Drawing for the job (mm, zero at the part's lowest x, y, z). Coordinates: 2 decimals unless noted, no trailing zeros. Loops run counter-clockwise (first coordinate to the right, second up) from the corner with the lowest first, then second, coordinate; pieces in that order, holes last. Notation, with made-up numbers: (27.5, 85.25) - (69.5, 85.25) arc R11 cw to (69.5, 106.25) - close; hole circle Ø1 at (35.5, 35.5). An arc over 180 degrees is marked (long way). Put each result on its own line as item: value.
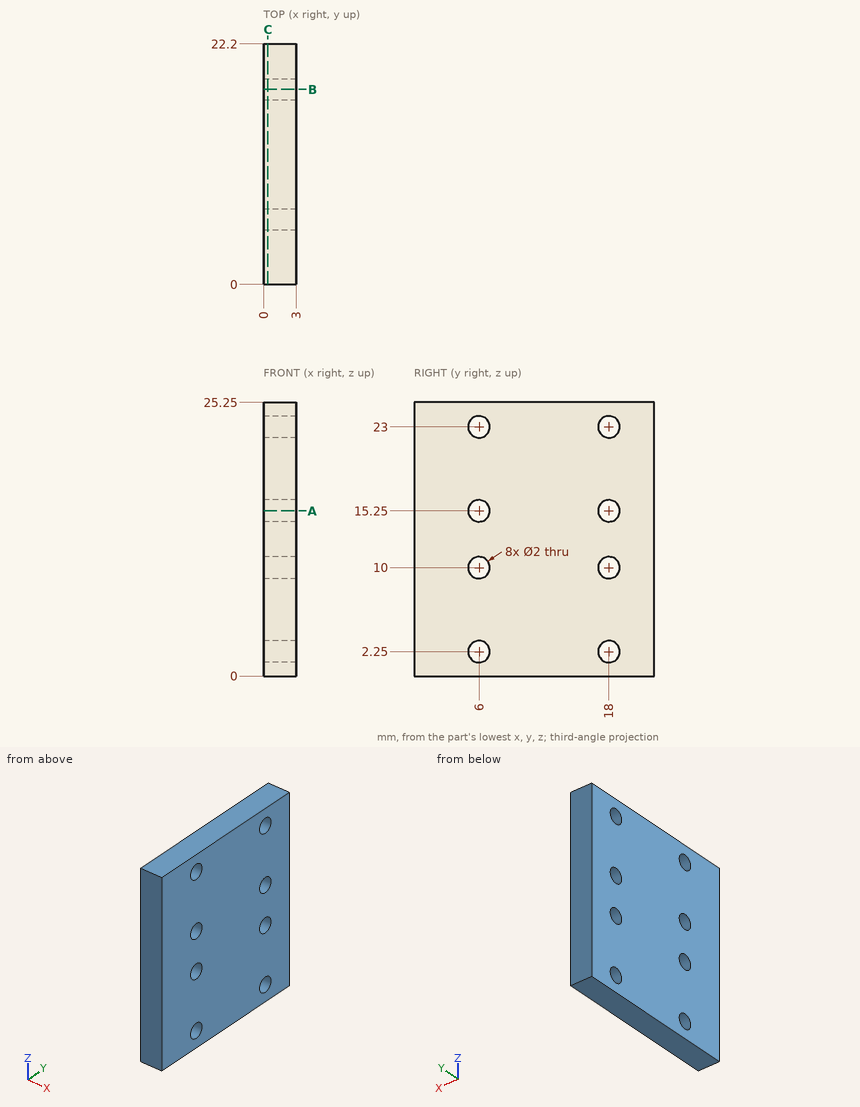
Q1. Slice it at B-B, the plane y = 18. Give the cut face in (x, z).
Determined:
outline: (0, 0) - (3, 0) - (3, 1.25) - (0, 1.25) - close; (0, 3.25) - (3, 3.25) - (3, 9) - (0, 9) - close; (0, 11) - (3, 11) - (3, 14.25) - (0, 14.25) - close; (0, 16.25) - (3, 16.25) - (3, 22) - (0, 22) - close; (0, 24) - (3, 24) - (3, 25.25) - (0, 25.25) - close
Q2. Pin check, flat tip, straight feed: pin 1 Ø1.2 at (y, z) = (6, 15.25) entering from -X. Stop position of the tip, or through.
Determined:
pin 1: through
Q3. Slice it at A-A, the plane z = 15.25. Give the cut face in (x, y).
Determined:
outline: (0, 0) - (3, 0) - (3, 5) - (0, 5) - close; (0, 7) - (3, 7) - (3, 17) - (0, 17) - close; (0, 19) - (3, 19) - (3, 22.2) - (0, 22.2) - close
Q4. Wall check: L1, parallel to Z at x = 2.35, y = 18; L2, parallel to Y at x = 1, z = 22.75; L3, parallel to Z at x = 2.45, y = 6.75. Give the ranges that are in metal, low to high. Write a range as from..to.
Determined:
L1: 0..1.25, 3.25..9, 11..14.25, 16.25..22, 24..25.25
L2: 0..5.03, 6.97..17.03, 18.97..22.2
L3: 0..1.59, 2.91..9.34, 10.66..14.59, 15.91..22.34, 23.66..25.25
Q5. Slice it at C-C, the plane x = 0.4. State how many separate pieces and enclosed holes the cut face has, then the cut area to 3 significant figures.
Determined:
separate pieces: 1
enclosed holes: 8
area: 535 mm2
